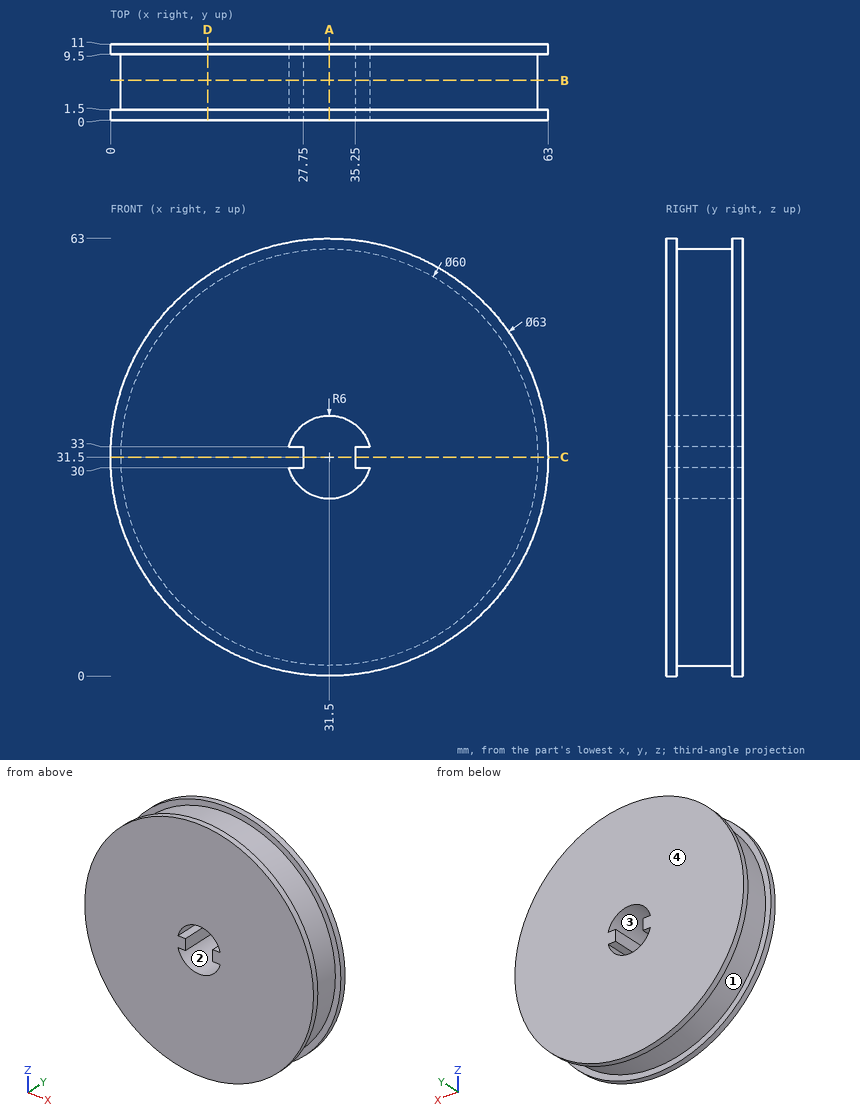
The drawing under review shows one solid part. Ordinate dimensions are in mm from its lowest x, y, z. Round coordinates to 2 decimals unless told otherwise and drop trailing zeros. Write each loop counter-clockwise with the first axis right and the second up, starting at its lowest first coordinate (ties: lowest second). Pieces come first, ordered by that corner, then holes. Notation, with made-up numbers: (54, -26) - (86, -26) arc R19 cw to (86, 10) - close; hole circle Ø6 at (-23.5, 57.25). An arc over 180 degrees is marked (long way). Put each result on its own line as item: value.
Q1. Insertion check: pin 1 Ø4 at (y, z) = (9.5, 19.5) entering from -X; pin 2 Ø0.6 at (x, y) = (36, 6.5) entering from -Z; pin 3 Ø0.9 at (y, z) = (7, 31) entering from +X. Each pin has a flat end and moves straight along its axis. Give the tip position at first contact, or say it passes through.
Solved:
pin 1: stops at x = 1.63
pin 2: stops at z = 1.8
pin 3: stops at x = 61.5
Q2. Wall thickness on probe 1 along Y at (x, z) = (5, 48); probe 2 along X at (y, z) = (4.75, 34); probe 3 along X at (y, z) = (7, 52): over which ranges is each line inside the solid? List them lowest first.
Solved:
probe 1: y = 0 to 1.5, 9.5 to 11
probe 2: x = 1.6 to 26.05, 36.95 to 61.4
probe 3: x = 9.6 to 53.4
Q3. Mouldability with a two-part tool opening along Z and no side actions: class the marked faces 1, 2, 3 and 4 as released by +Z, released by -Z, zero draft, split by the parting line, or undercut.
Solved:
face 1: split by the parting line
face 2: undercut
face 3: undercut
face 4: zero draft
Q4. We need section B-B (y = 5.75). Give the boundary of the cut face in (x, z).
Solved:
outline: circle Ø60 at (31.5, 31.5); hole (25.69, 30) arc R6 ccw to (37.31, 30) - (35.25, 30) - (35.25, 33) - (37.31, 33) arc R6 ccw to (25.69, 33) - (27.75, 33) - (27.75, 30) - close
Q5. We need section A-A (x = 31.5). Give the boundary of the cut face in (y, z), and give its area (3 significant figures).
Solved:
outline: (0, 0) - (1.5, 0) - (1.5, 1.5) - (9.5, 1.5) - (9.5, 0) - (11, 0) - (11, 25.5) - (0, 25.5) - close; (0, 37.5) - (11, 37.5) - (11, 63) - (9.5, 63) - (9.5, 61.5) - (1.5, 61.5) - (1.5, 63) - (0, 63) - close
area: 537 mm2
Q6. We need section C-C (z = 31.5). Give the boundary of the cut face in (x, y), and give its area (4 significant figures).
Solved:
outline: (0, 0) - (27.75, 0) - (27.75, 11) - (0, 11) - (0, 9.5) - (1.5, 9.5) - (1.5, 1.5) - (0, 1.5) - close; (35.25, 0) - (63, 0) - (63, 1.5) - (61.5, 1.5) - (61.5, 9.5) - (63, 9.5) - (63, 11) - (35.25, 11) - close
area: 586.5 mm2
Q7. We need section D-D (x = 14). Give the boundary of the cut face in (y, z), and give its area (3 significant figures).
Solved:
outline: (0, 5.31) - (1.5, 5.31) - (1.5, 7.13) - (9.5, 7.13) - (9.5, 5.31) - (11, 5.31) - (11, 57.69) - (9.5, 57.69) - (9.5, 55.87) - (1.5, 55.87) - (1.5, 57.69) - (0, 57.69) - close
area: 547 mm2
